Read the model definition and answer for the solid it produces. Units are mm, in the model's axes. A direction names the side the tool comes from. Round coordinates to 2 decimals unless told otherwise and drop trailing zeros. Order: outer loops, then holes, each group sorted by start corner. A loop starts at its lowest first (then second) coordinate and runs counter-clockwise, first axis right, second up. Notation, with made-up numbers: (81, -12) - (98, -12) arc R29 cw to (98, 10) - close; hole circle Ø5 at (-33, -35). An arc over 180 degrees is marked (long way). Answer as a JSON object with one key per item and string values. Group by question number.
Q1. Consider line 1 (Y direction, x = 20, z = 20); line 2 (Z direction, x = 23, y = 9); line 3 (Y direction, x = -6, z = -6.5). Determine where each line is inside the solid, lowest interval first.
Q2. Given pin 1 Ø13.5 at (x, y) = (0, 0) entering from +Z; pin 2 Ø3 at (x, z) = (23, 21.5) entering from +Y; pin 3 Ø3 at (x, z) = (7.5, -8.5) entering from -Y; pin 4 Ø1.5 at (y, z) = (-10, -2) entering from +X, each flat-ended and moving along its own axis, determine where each tip first touches the part or whether it passes through.
Q3. A cutting plane is placed at B-B on z = 23. Determine the outline of the cut face in (x, y).
Q4. A cutting plane is placed at D-D on y = 35. Determine the outline of the cut face in (x, z), and give its area (3 significant figures).
Q5. A cutting plane is placed at C-C on z = 35. Determine the outline of the cut face in (x, y), and give its area (3 significant figures).
Q6. The mould has two halves that part along Z. Classify faces 5 (the flat face through (0, -17.5, 15)), 6 (the cylindrical face through (0.21, 43.07, 13.4)), 7 (the flat face through (0, 47, 40)): pulls with the +Z half, pulls with the -Z half, needs draft (parallel to the pull), parting line crosses it, or undercut.
Q7. A cutting plane is placed at A-A on x = 8. Determine the outline of the cut face in (y, z), and give its area (3 significant figures).
Q8. A tool of negligible diameter and unlimited length cuts with its end or side. For faces 1 (the cylindrical face through (-12.503, 0.226, 14.804)), 2 (the flat face through (-23, 17.5, 15)), 3 (the flat face through (2, -4, 19)), 4 (the flat face through (-4, 31, 17)), from which of +Z, -Z, +X, -X, +Y, -Y can it reach the whole face along a straight path? Write none if from no direction.
```python
from build123d import *

# Parameters (mm, degrees)
SKETCH_1_W              = 50
SKETCH_1_H              = 35
EXTRUDE_1_DEPTH         = 30
HOLE_WIZARD_360_D       = 8.5
HOLE_WIZARD_465_D       = 3.2
HOLE_WIZARD_619_D       = 15
CHAMFER_1_SIZE          = 1
CHAMFER_1_SIZE_2        = 0.708203932
SKETCH_8_W              = 15
SKETCH_8_H              = 15
EXTRUDE_2_DEPTH         = 35
HOLE_WIZARD_1775_D      = 10.4
HOLE_WIZARD_1775_DEPTH  = 11
HOLE_WIZARD_1887_D      = 10.4
HOLE_WIZARD_1887_DEPTH  = 11
HOLE_WIZARD_2064_D      = 8.5
CUT_EXTRUDE_START       = -40
CUT_EXTRUDE_1_OUTLINE_R = 1.6
CUT_EXTRUDE_1_DEPTH     = 30
CHAMFER_2_SIZE          = 1
CHAMFER_2_SIZE_2        = 0.708203933
RIB_START               = -15
RIB_8_DEPTH             = 30
RIB_10_REACH            = 72.578
SKETCH_20_WALL_W        = 151.64122351
SKETCH_20_WALL_H        = 30


with BuildPart() as part:
    # 草图1 → 凸台-拉伸1 (new body)
    with BuildSketch(Plane.XY):
        Rectangle(SKETCH_1_W, SKETCH_1_H)
    extrude(amount=EXTRUDE_1_DEPTH)

    # Hole Wizard 360 (through all)
    with Locations(Plane.XY.offset(30)):
        with Locations((0, 0)):
            Hole(HOLE_WIZARD_360_D / 2)

    # Hole Wizard 465 (through all)
    with Locations(Plane.XY.offset(30)):
        with Locations((8, 0), (0, 8), (-8, 0), (0, -8)):
            Hole(HOLE_WIZARD_465_D / 2)

    # Hole Wizard 619 (through all)
    with Locations(Plane.XY.offset(30)):
        with Locations((20, 0), (-20, 0)):
            Hole(HOLE_WIZARD_619_D / 2)

    # 倒角1
    # the kernel refuses this chamfer: 1, 0.708203932 mm, written as the material it takes off along each edge
    with BuildSketch(Plane(origin=(-20, 0, 0), x_dir=(-0.8790200859122482, 0.4767847402789059, 0), z_dir=(-0.4767847402789059, -0.8790200859122482, 0))) as chamfer_1_piece_1:
        Polygon((7.5, -CHAMFER_1_SIZE), (7.5 + CHAMFER_1_SIZE, 0), (7.5, 0), align=None)
    revolve(axis=Axis((-20, 0, 0), (0, 0, -1)), revolution_arc=303.048763938, mode=Mode.SUBTRACT)
    with BuildSketch(Plane(origin=(-20, 0, 30), x_dir=(-0.879020085912248, 0.47678474027890627, 0), z_dir=(-0.47678474027890627, -0.879020085912248, 0))) as chamfer_1_piece_2:
        Polygon((7.5 + CHAMFER_1_SIZE, 0), (7.5, CHAMFER_1_SIZE), (7.5, 0), align=None)
    revolve(axis=Axis((-20, 0, 30), (0, 0, -1)), revolution_arc=303.048763938, mode=Mode.SUBTRACT)
    with BuildSketch(Plane(origin=(20, 0, 30), x_dir=(0.879020085912248, -0.4767847402789061, 0), z_dir=(0.4767847402789061, 0.879020085912248, 0))) as chamfer_1_piece_3:
        Polygon((7.5 + CHAMFER_1_SIZE, 0), (7.5, CHAMFER_1_SIZE), (7.5, 0), align=None)
    revolve(axis=Axis((20, 0, 30), (0, 0, -1)), revolution_arc=303.048763938, mode=Mode.SUBTRACT)
    with BuildSketch(Plane(origin=(20, 0, 0), x_dir=(0.8790200859122481, 0.476784740278906, 0), z_dir=(0.476784740278906, -0.8790200859122481, 0))) as chamfer_1_piece_4:
        Polygon((7.5, CHAMFER_1_SIZE), (7.5 + CHAMFER_1_SIZE, 0), (7.5, 0), align=None)
    revolve(axis=Axis((20, 0, 0), (0, 0, 1)), revolution_arc=303.048763938, mode=Mode.SUBTRACT)
    with BuildSketch(Plane(origin=(-25, 5.590169944, 32.778051389), x_dir=(0.7914486393779661, 0.611235675682274, 0), z_dir=(0, 0, -1)), Plane(origin=(25, -5.590169944, 32.778051389), x_dir=(-0.7914486393779661, -0.611235675682274, 0), z_dir=(0, 0, -1))) as chamfer_1_piece_5:
        with BuildLine():
            Line((1.080663788, 0), (CHAMFER_1_SIZE_2 * 0.611235676113, -CHAMFER_1_SIZE_2 * 0.791448639936))
            Line((CHAMFER_1_SIZE_2 * 0.611235676113, -CHAMFER_1_SIZE_2 * 0.791448639936), (0, 0))
            ThreePointArc((0, 0), (0.555522087, -0.019473843), (1.080663788, 0))
        make_face()
    extrude(amount=35.556102778, mode=Mode.SUBTRACT)
    with BuildSketch(Plane(origin=(-25, -5.590169944, 32.778051389), x_dir=(0.7914486393779665, -0.6112356756822735, 0), z_dir=(0, 0, -1))) as chamfer_1_piece_6:
        with BuildLine():
            Line((1.080663788, 0), (CHAMFER_1_SIZE_2 * 0.611235676113, CHAMFER_1_SIZE_2 * 0.791448639936))
            Line((CHAMFER_1_SIZE_2 * 0.611235676113, CHAMFER_1_SIZE_2 * 0.791448639936), (0, 0))
            ThreePointArc((0, 0), (0.555522087, 0.019473843), (1.080663788, 0))
        make_face()
    extrude(amount=35.556102778, mode=Mode.SUBTRACT)
    with BuildSketch(Plane(origin=(25, 5.590169944, 32.778051389), x_dir=(0, 1, 0), z_dir=(0, 0, -1))) as chamfer_1_piece_7:
        with BuildLine():
            Line((CHAMFER_1_SIZE_2, 0), (0.660540261, -0.855289885))
            ThreePointArc((0.660540261, -0.855289885), (0.354967464, -0.427764092), (0, 0))
            Line((0, 0), (CHAMFER_1_SIZE_2, 0))
        make_face()
    extrude(amount=35.556102778, mode=Mode.SUBTRACT)

    # 草图8 → 凸台-拉伸2 (add)
    with BuildSketch(Plane(origin=(0, 17.5, 0), x_dir=(1, 0, 0), z_dir=(0, 1, 0))):
        Polygon((15, -30), (0, -30), (-15, -30), (-15, -40), (15, -40), align=None)
        with Locations((-7.5, -22.5)):
            Rectangle(SKETCH_8_W, SKETCH_8_H)
        with Locations((-7.5, -7.5)):
            Rectangle(SKETCH_8_W, SKETCH_8_H)
        Polygon((-15, 0), (0, 0), (15, 0), (15, 10), (-15, 10), align=None)
        with Locations((7.5, -7.5)):
            Rectangle(SKETCH_8_W, SKETCH_8_H)
        with Locations((7.5, -22.5)):
            Rectangle(SKETCH_8_W, SKETCH_8_H)
    extrude(amount=EXTRUDE_2_DEPTH)

    # Hole Wizard 1775
    with Locations(Plane.XY.offset(30)):
        with Locations((0, 0)):
            Hole(HOLE_WIZARD_1775_D / 2, depth=HOLE_WIZARD_1775_DEPTH)

    # Hole Wizard 1887
    with Locations(Plane.ZY.offset(15)):
        with Locations((15, 35)):
            Hole(HOLE_WIZARD_1887_D / 2, depth=HOLE_WIZARD_1887_DEPTH)

    # Hole Wizard 2064 (through all)
    with Locations(Plane.ZY.offset(15)):
        with Locations((15, 35)):
            Hole(HOLE_WIZARD_2064_D / 2)

    # 切除-拉伸1: read off the stored shape, not the designer's step
    # 切除-拉伸1 outline → 切除-拉伸1 (cut)
    with BuildSketch(Plane.ZY.offset(25).offset(CUT_EXTRUDE_START)):
        with Locations((23, 35)):
            Circle(CUT_EXTRUDE_1_OUTLINE_R)
        with Locations((7, 35)):
            Circle(CUT_EXTRUDE_1_OUTLINE_R)
        with Locations((15, 43)):
            Circle(CUT_EXTRUDE_1_OUTLINE_R)
        with BuildLine():
            Line((40, 29.409830056), (40, 40.590169944))
            ThreePointArc((40, 40.590169944), (27.5, 35), (40, 29.409830056))
        make_face()
        with Locations((15, 27)):
            Circle(CUT_EXTRUDE_1_OUTLINE_R)
        with BuildLine():
            Line((-10, 40.590169944), (-10, 29.409830056))
            ThreePointArc((-10, 29.409830056), (2.5, 35), (-10, 40.590169944))
        make_face()
    extrude(amount=CUT_EXTRUDE_1_DEPTH, mode=Mode.SUBTRACT)

    # 倒角2
    # the kernel refuses this chamfer: 1, 0.708203933 mm, written as the material it takes off along each edge
    with BuildSketch(Plane(origin=(-15, 35, 35), x_dir=(0, 0.4767847403128172, 0.8790200858938546), z_dir=(0, -0.8790200858938546, 0.4767847403128172))) as chamfer_2_piece_1:
        Polygon((7.5 + CHAMFER_2_SIZE, 0), (7.5, -CHAMFER_2_SIZE), (7.5, 0), align=None)
    revolve(axis=Axis((-15, 35, 35), (-1, 0, 0)), revolution_arc=303.048763934, mode=Mode.SUBTRACT)
    with BuildSketch(Plane(origin=(-15, 35, -5), x_dir=(0, -0.4767847403128172, -0.8790200858938546), z_dir=(0, 0.8790200858938546, -0.4767847403128172))) as chamfer_2_piece_2:
        Polygon((7.5 + CHAMFER_2_SIZE, 0), (7.5, -CHAMFER_2_SIZE), (7.5, 0), align=None)
    revolve(axis=Axis((-15, 35, -5), (-1, 0, 0)), revolution_arc=303.048763934, mode=Mode.SUBTRACT)
    with BuildSketch(Plane(origin=(15, 35, -5), x_dir=(0, -0.4767847403128172, -0.8790200858938546), z_dir=(0, 0.8790200858938546, -0.4767847403128172))) as chamfer_2_piece_3:
        Polygon((7.5 + CHAMFER_2_SIZE, 0), (7.5, CHAMFER_2_SIZE), (7.5, 0), align=None)
    revolve(axis=Axis((15, 35, -5), (-1, 0, 0)), revolution_arc=303.048763934, mode=Mode.SUBTRACT)
    with BuildSketch(Plane(origin=(15, 35, 35), x_dir=(0, 0.4767847403128172, 0.8790200858938546), z_dir=(0, -0.8790200858938546, 0.4767847403128172))) as chamfer_2_piece_4:
        Polygon((7.5 + CHAMFER_2_SIZE, 0), (7.5, CHAMFER_2_SIZE), (7.5, 0), align=None)
    revolve(axis=Axis((15, 35, 35), (-1, 0, 0)), revolution_arc=303.048763934, mode=Mode.SUBTRACT)
    with BuildSketch(Plane(origin=(17.778051389, 40.590169944, -10), x_dir=(0, 0.6112356756567692, 0.7914486393976635), z_dir=(-1, 0, 0))) as chamfer_2_piece_5:
        with BuildLine():
            Line((1.080663788, 0), (CHAMFER_2_SIZE_2 * 0.611235675226, CHAMFER_2_SIZE_2 * 0.79144863884))
            Line((CHAMFER_2_SIZE_2 * 0.611235675226, CHAMFER_2_SIZE_2 * 0.79144863884), (0, 0))
            ThreePointArc((0, 0), (0.555522087, 0.019473843), (1.080663788, 0))
        make_face()
    extrude(amount=35.556102778, mode=Mode.SUBTRACT)
    with BuildSketch(Plane(origin=(17.778051389, 29.409830056, -10), x_dir=(0, -1, 0), z_dir=(-1, 0, 0)), Plane(origin=(17.778051389, 40.590169944, 40), x_dir=(0, 1, 0), z_dir=(-1, 0, 0))) as chamfer_2_piece_6:
        with BuildLine():
            Line((CHAMFER_2_SIZE_2, 0), (0.660540261, 0.855289885))
            ThreePointArc((0.660540261, 0.855289885), (0.354967464, 0.427764092), (0, 0))
            Line((0, 0), (CHAMFER_2_SIZE_2, 0))
        make_face()
    extrude(amount=35.556102778, mode=Mode.SUBTRACT)
    with BuildSketch(Plane(origin=(17.778051389, 29.409830056, 40), x_dir=(0, -1, 0), z_dir=(-1, 0, 0))) as chamfer_2_piece_7:
        with BuildLine():
            Line((CHAMFER_2_SIZE_2, 0), (0.660540261, -0.855289885))
            ThreePointArc((0.660540261, -0.855289885), (0.354967464, -0.427764092), (0, 0))
            Line((0, 0), (CHAMFER_2_SIZE_2, 0))
        make_face()
    extrude(amount=35.556102778, mode=Mode.SUBTRACT)

    # 筋8: read off the stored shape, not the designer's step
    # 筋8 outline → 筋8 (add)
    with BuildSketch(Plane.XY.offset(15).offset(RIB_START)):
        Polygon((21, 17.5), (15, 23.5), (15, 17.5), align=None)
    rib_8 = extrude(amount=RIB_8_DEPTH)

    # 镜向3: 筋8 across plane
    add(rib_8.mirror(Plane.ZY))

    # 草图20 wall → 筋10 (add, up to next)
    with BuildSketch(Plane(origin=(0, 14.5, 33), x_dir=(0, -0.707106781187, -0.707106781187), z_dir=(0, -0.707106781187, 0.707106781187)), mode=Mode.PRIVATE) as rib_10_sk1:
        Rectangle(SKETCH_20_WALL_W, SKETCH_20_WALL_H)
    rib_10_tool1 = extrude(rib_10_sk1.sketch, amount=-RIB_10_REACH, mode=Mode.PRIVATE) - part.part
    rib_10 = rib_10_tool1.solids().sort_by_distance((0, 14.5, 33))[0]
    add(rib_10)

    # 镜向4: 筋10 across plane
    add(rib_10.mirror(Plane.XY.offset(15)))


solid = part.part
```
Result set:
{
 "1": {"line 1": "y = -17.5 to -7.5, 7.5 to 18.5", "line 2": "z = 0 to 30", "line 3": "y = 17.5 to 27.65, 42.35 to 52.5"},
 "2": {"pin 1": "stops at z = 30", "pin 2": "stops at y = 17.5", "pin 3": "stops at y = 17.5", "pin 4": "passes through"},
 "3": {"outline": "(-25, -17.5) - (25, -17.5) - (25, -6.3) - (24.14, -6.25) arc R7.5 cw (long way) to (24.14, 6.25) - (25, 6.3) - (25, 17.5) - (21, 17.5) - (15, 23.5) - (15, 33.4) - (-15, 33.4) - (-15, 23.5) - (-21, 17.5) - (-25, 17.5) - (-25, 6.3) - (-24.14, 6.25) arc R7.5 cw (long way) to (-24.14, -6.25) - (-25, -6.3) - close; (-15, 36.6) - (15, 36.6) - (15, 52.5) - (-15, 52.5) - close; hole circle Ø3.2 at (-8, 0); hole circle Ø10.4 at (0, 0); hole circle Ø3.2 at (0, -8); hole circle Ø3.2 at (0, 8); hole circle Ø3.2 at (8, 0)"},
 "4": {"outline": "(-15, 3.5) - (-14, 2.5) - (14, 2.5) - (15, 3.5) - (15, 5.4) - (-15, 5.4) - close; (-15, 8.6) - (15, 8.6) - (15, 10.75) - (-4, 10.75) - (-4, 9.8) - (-15, 9.8) - close; (-15, 20.2) - (-4, 20.2) - (-4, 19.25) - (15, 19.25) - (15, 21.4) - (-15, 21.4) - close; (-15, 24.6) - (15, 24.6) - (15, 26.5) - (14, 27.5) - (-14, 27.5) - (-15, 26.5) - close", "area": "280 mm²"},
 "5": {"outline": "(-15, 16.5) - (15, 16.5) - (15, 26.5) - (14, 27.5) - (-14, 27.5) - (-15, 26.5) - close; (-15, 43.5) - (-14, 42.5) - (14, 42.5) - (15, 43.5) - (15, 52.5) - (-15, 52.5) - close", "area": "628 mm²"},
 "6": {"face 5": "needs draft", "face 6": "undercut", "face 7": "pulls with the +Z half"},
 "7": {"outline": "(-17.5, 0) - (-1.6, 0) - (-1.6, 30) - (-17.5, 30) - close; (1.6, 0) - (11.5, 0) - (17.5, -6) - (17.5, -10) - (28.7, -10) - (28.75, -9.14) arc R7.5 cw (long way) to (41.25, -9.14) - (41.3, -10) - (52.5, -10) - (52.5, 40) - (41.3, 40) - (41.25, 39.14) arc R7.5 cw (long way) to (28.75, 39.14) - (28.7, 40) - (17.5, 40) - (17.5, 36) - (11.5, 30) - (1.6, 30) - close; hole circle Ø3.2 at (27, 15); hole circle Ø8.5 at (35, 15); hole circle Ø3.2 at (35, 7); hole circle Ø3.2 at (35, 23); hole circle Ø3.2 at (43, 15)", "area": "2,340 mm²"},
 "8": {"face 1": "+Z, -Z", "face 2": "+Z, -Z, -X, +Y", "face 3": "+Z", "face 4": "-X"}
}
